Could you check a few things on this model? Use its own coordinates, in mm. A direction names the side the tool comes from. Round coordinates to 2 decimals unless told otherwise and drop trailing zeros. Loops run counter-clockwise (first coordinate to the right, second up) from the corner with the lowest first, then second, coordinate; pieces in that order, holes last. Notation, with made-up numbers: (-13.5, -12.5) -> (-4.5, -12.5) arc R13 cw to (-4.5, 3.5) -> close; hole circle Ø1 at (30.25, -20.75). An arc over 180 degrees is marked (long way). Put each result on its own line as item: value. Start each with the question number.
1. Imagine slicing it at C-C, the plane z = -1275. Please give me the cut outline in (x, y), and give its area (3 significant figures).
2. Imagine slicing it at A-A, the plane x = 0. Please give me the cut outline in (y, z), and give its area (3 significant figures).
3. I need wall thicknesses on line 1 (X direction, y = -69.5, z = -616); line 2 (Y direction, x = -78, z = -991.5); line 3 (X direction, y = 96.5, z = -957). Which ranges of each line are inside material? Lowest first, please. Write a range as [from, to].
4. Which directions (+Z, -Z, +X, -X, +Y, -Y) give clear straight access to the entire face, cutting with the end or side of a thin tool? Please do faces 4 (the flat face through (-2, 2, 0)), 5 (the flat face through (-35, 120, -1377)).
5. If we mould it in two halves opening along X, with no side actions, what happens to faces 1 (the cylindrical face through (-32.517, -146.433, -739.5)), 2 (the flat face through (0, 94.4, -1377)), 3 (the flat face through (-2, 0, -1500))? For each: pulls with the +X half, pulls with the -X half, needs draft (parallel to the pull), parting line crosses it, or undercut.
6. I'm going to push flat-ended pins straight in: P1, Ø8, axis at x = 36.5, z = -613.5, coming from the -Y side; P2, Ø2, axis at y = -104.5, z = -331, coming from the +X side; P3, Ø1, axis at y = -13.5, z = -346.5, coming from the +X side; P4, Ø1, axis at x = -47.5, y = 48.5, coming from the +Z side. Where does each tip first touch, or does it pass through?
7. Imagine slicing it at B-B, the plane y = -27. Please give me the cut outline in (x, z), and give its area (3 significant figures).
```python
from build123d import *

# Parameters (mm, degrees)
SKETCH1_R           = 150
BOSS_EXTRUDE1_DEPTH = 1500
SKETCH3_W           = 70
SKETCH3_H           = 70
CUT_EXTRUDE2_DEPTH  = 250
SKETCH7_R           = 150
SKETCH7_R_2         = 149.9999
EXTRUDE_THIN1_DEPTH = 92.5
EXTRUDE_THIN2_START = -74
SKETCH8_R           = 150
SKETCH8_R_2         = 149.9999
EXTRUDE_THIN2_DEPTH = 74


with BuildPart() as part:
    # Sketch1 → Boss-Extrude1 (new body)
    with BuildSketch(Plane.XY):
        Circle(SKETCH1_R)
    extrude(amount=-BOSS_EXTRUDE1_DEPTH)

    # Sketch3 → Cut-Extrude2 (cut)
    with BuildSketch(Plane(origin=(0, 0, -1500), x_dir=(-1, 0, 0), z_dir=(0, 0, -1))):
        with Locations((0, 129.4)):
            Rectangle(SKETCH3_W, SKETCH3_H)
    extrude(amount=-CUT_EXTRUDE2_DEPTH, mode=Mode.SUBTRACT)

    # Sketch7 → Extrude-Thin1 (add, symmetric)
    with BuildSketch(Plane.XY.offset(-400)):
        Circle(SKETCH7_R)
        Circle(SKETCH7_R_2, mode=Mode.SUBTRACT)
    extrude(amount=EXTRUDE_THIN1_DEPTH, both=True)

    # Sketch8 → Extrude-Thin2 (add)
    with BuildSketch(Plane(origin=(0, 0, -1200), x_dir=(-1, 0, 0), z_dir=(0, 0, -1)).offset(EXTRUDE_THIN2_START)):
        Circle(SKETCH8_R)
        Circle(SKETCH8_R_2, mode=Mode.SUBTRACT)
    extrude(amount=EXTRUDE_THIN2_DEPTH)


solid = part.part
```
Entries:
1. outline: (-35, 94.4) -> (-35, 145.86) arc R150 ccw (long way) to (35, 145.86) -> (35, 94.4) -> close
1. area: 66,900 mm^2
2. outline: (-150, -1500) -> (94.4, -1500) -> (94.4, -1250) -> (150, -1250) -> (150, 0) -> (-150, 0) -> close
2. area: 436,000 mm^2
3. line 1: [-132.93, 132.93]
3. line 2: [-128.12, 128.12]
3. line 3: [-114.84, 114.84]
4. face 4: +Z, +X, -X, +Y, -Y
4. face 5: -Z, +Y
5. face 1: parting line crosses it
5. face 2: undercut
5. face 3: needs draft
6. P1: y = -146.44
6. P2: x = 108.57
6. P3: x = 149.44
6. P4: z = 0
7. outline: (-147.55, -1500) -> (147.55, -1500) -> (147.55, 0) -> (-147.55, 0) -> close
7. area: 443,000 mm^2
